```python
from build123d import *

# Parameters (mm, degrees)
F0_W      = 42
F0_H      = 42
F1_DEPTH  = 44
F2_R      = 11
F3_DEPTH  = 2
F4_R      = 2.5
F5_DEPTH  = 20
F6_R      = 2.5
F7_DEPTH  = 10
F8_W      = 17
F8_H      = 9.8
F9_DEPTH  = 1.5
F10_R     = 5
F11_R     = 3
F12_W     = 15
F12_H     = 5.6
F13_DEPTH = 1
F14_W     = 15
F14_H     = 5.6
F14_W_2   = 13
F14_H_2   = 3.6
F15_DEPTH = 4
F16_W     = 0.5
F16_H     = 0.5
F17_DEPTH = 4
F18_R     = 0.49999
F19_W     = 10
F19_H     = 1
F20_DEPTH = 3.5


# Not quite as in the source:
# - a fillet or chamfer is up to 0.001 mm smaller than in the source, because OpenCascade refuses the exact size


with BuildPart() as f1:
    # F0 (on Front) → F1 (new body)
    with BuildSketch(Plane.XZ):
        Rectangle(F0_W, F0_H)
    extrude(amount=F1_DEPTH)

    # F2 (on face) → F3 (join)
    with BuildSketch(Plane.XZ.offset(44)):
        Circle(F2_R)
    extrude(amount=F3_DEPTH)

    # F4 (on face) → F5 (join)
    with BuildSketch(Plane.XZ.offset(46)):
        Circle(F4_R)
    extrude(amount=F5_DEPTH)

    # F6 (on face) → F7 (cut)
    with BuildSketch(Plane.XZ.offset(44)):
        with Locations((-15.5, 15.5)):
            Circle(F6_R)
        with Locations((15.5, 15.5)):
            Circle(F6_R)
        with Locations((15.5, -15.5)):
            Circle(F6_R)
        with Locations((-15.5, -15.5)):
            Circle(F6_R)
    extrude(amount=-F7_DEPTH, mode=Mode.SUBTRACT)

    # F8 (on face) → F9 (join)
    with BuildSketch(Plane.XY.offset(21)):
        with Locations((0, -4.9)):
            Rectangle(F8_W, F8_H)
    extrude(amount=F9_DEPTH)

    # F10
    f10_edges = [f1.edges().sort_by_distance(p)[0] for p in [
        (-21, -22, 21),
        (21, -22, 21),
        (21, -22, -21),
        (-21, -22, -21),
    ]]
    fillet(f10_edges, radius=F10_R)

    # F11
    f11_edges = [f1.edges().sort_by_distance(p)[0] for p in [
        (12.25, 0, 21),
        (19.535534, 0, 19.535534),
        (8.5, 0, 21.75),
        (21, 0, 0),
        (0, 0, 22.5),
        (19.535534, 0, -19.535534),
        (-8.5, 0, 21.75),
        (0, 0, -21),
        (-12.25, 0, 21),
        (-19.535534, 0, -19.535534),
        (-19.535534, 0, 19.535534),
        (-21, 0, 0),
    ]]
    fillet(f11_edges, radius=F11_R)

    # F12 (on face) → F13 (join)
    with BuildSketch(Plane.XY.offset(22.5)):
        with Locations((0, -6.5)):
            Rectangle(F12_W, F12_H)
    extrude(amount=F13_DEPTH)

    # F14 (on face) → F15 (join)
    with BuildSketch(Plane.XY.offset(23.5)):
        with Locations((0, -6.5)):
            Rectangle(F14_W, F14_H)
        with Locations((0, -6.5)):
            Rectangle(F14_W_2, F14_H_2, mode=Mode.SUBTRACT)
    extrude(amount=F15_DEPTH)

    # F16 (on face) → F17 (join)
    with BuildSketch(Plane.XY.offset(23.5)):
        with Locations((-5.417, -6.5)):
            Rectangle(F16_W, F16_H)
        with Locations((-3.25, -6.5)):
            Rectangle(F16_W, F16_H)
        with Locations((-1.083, -6.5)):
            Rectangle(F16_W, F16_H)
        with Locations((3.25, -6.5)):
            Rectangle(F16_W, F16_H)
        with Locations((1.083, -6.5)):
            Rectangle(F16_W, F16_H)
        with Locations((5.417, -6.5)):
            Rectangle(F16_W, F16_H)
    extrude(amount=F17_DEPTH)

    # F18 (radius 0.5 in the source; OpenCascade refuses exactly that, so slightly less here)
    f18_edges = [f1.edges().sort_by_distance(p)[0] for p in [
        (0, -9.8, 22.5),
        (8.5, -9.8, 21.75),
        (8.5, -6.4, 22.5),
        (-8.5, -9.8, 21.75),
        (-8.5, -6.4, 22.5),
        (-7.438147, -0.710112, 21.438147),
        (7.438147, -0.710112, 21.438147),
        (0, 0, 19.5),
        (5.5, 0, 18.75),
        (-5.5, 0, 18.75),
    ]]
    fillet(f18_edges, radius=F18_R)

    # F19 (on face) → F20 (cut)
    with BuildSketch(Plane.XY.offset(27.5)):
        with Locations((0, -8.8)):
            Rectangle(F19_W, F19_H)
    extrude(amount=-F20_DEPTH, mode=Mode.SUBTRACT)


solid = f1.part
```
CAD build for the part. Positions are in the model's coordinates, mm. A direction names the side the tool comes from. Give positions to 0.01 mm unless a question says otherwise; leave off trailing zeros. Loops run counter-clockwise (first coordinate to the right, second up) from the corner with the lowest first, then second, coordinate; pieces in that order, holes last. Notation, with made-up numbers: M 79.25,-30.75 L 87.25,-30.75 A17 ccw 87.25,-20.75 Z; hole C -3.75,8 d8. An arc over 180 degrees is marked long. Use one line per item in the form item = value.
Item 1: Slice it at A-A (z = 0). List the corners of the cut face in (x, y), plus the area to 3 significant figures.
Determined:
outline = M -21,-44 L -11,-44 L -11,-46 L -2.5,-46 L -2.5,-66 L 2.5,-66 L 2.5,-46 L 11,-46 L 11,-44 L 21,-44 L 21,-3 A3 ccw 18,0 L -18,0 A3 ccw -21,-3 Z
area = 1,990 mm2
Item 2: Slice it at D-D (z = 6). List the corners of the cut face in (x, y).
Determined:
outline = M -21,-44 L -9.22,-44 L -9.22,-46 L 9.22,-46 L 9.22,-44 L 21,-44 L 21,-3 A3 ccw 18,0 L -18,0 A3 ccw -21,-3 Z
Item 3: Drill centre lines: probe 1 along Z at (x, y) = (15.5, -36.25); probe 2 along X at (y, z) = (-37, 15); probe 3 along X at (y, z) = (-35.5, -14.5). Where is each one in solid material? Low to high. Write a range as from..to.
Determined:
probe_1 = -21..-18, -13..13, 18..21
probe_2 = -21..-17.95, -13.05..13.05, 17.95..21
probe_3 = -21..-17.79, -13.21..13.21, 17.79..21
Item 4: Two-plate mould, pull along X, no slides. Class faces 1 (the face through (-16, -34, -15)), 2 (the face through (19, -24, 20)), 3 (the face through (0, -66, 0)), 4 (the face through (-20, -24, -19)): pulls with the +X half, pulls with the -X half, needs draft (parallel to the pull), parting line crosses it, or undercut.
Determined:
face_1 = undercut
face_2 = pulls with the +X half
face_3 = needs draft
face_4 = pulls with the -X half
Item 5: Which spindle directions (+Z, -Z, +X, -X, +Y, -Y) get a long thin tool onto all of the face, cutting with end or side? Do faces 5 (the face through (-7.5, -7, 25)), 6 (the face through (0, -4.7, 25)), 7 (the face through (0, -9.3, 23)), 8 (the face through (7.35, -0.64, 20.45)). Say none if no direction does.
Determined:
face_5 = +Z, -X, +Y, -Y
face_6 = +Z
face_7 = +Z, +X, -X, -Y
face_8 = +Z, +X, +Y
Item 6: Slice it at C-C (y = -11). List the corners of the cut face in (x, z).
Determined:
outline = M -21,-16 A5 ccw -16,-21 L 16,-21 A5 ccw 21,-16 L 21,16 A5 ccw 16,21 L -16,21 A5 ccw -21,16 Z
Item 7: Flat gauge pins, fed straight in: pin 1 (4 mm diameter, centred on x = 0, z = 25, fed in from -Y); pin 2 (0.6 mm diameter, centred on x = -5.5, z = 26, fed in from +Y); pin 3 (1 mm diameter, centred on x = 2, z = 9, fed in from -Y). Where does each tip first touch, or does it go through?
Determined:
pin_1 = -9.3
pin_2 = -3.7
pin_3 = -46
